Autodesk Inventor part; units mm, degrees
ref_plane "YZ Plane" through (0, 0, 0) normal (1, 0, 0) x (0, 1, 0)
ref_plane "XZ Plane" through (0, 0, 0) normal (0, 1, 0) x (-1, 0, 0)
ref_plane "XY Plane" through (0, 0, 0) normal (0, 0, 1) x (1, 0, 0)
sketch "Sketch1" plane through (0, 0, 0) normal (0, 0, 1) x (1, 0, 0)
  line L0 (0, 0) -> (600, 0)
  line L1 (100, -188) -> (500, -188)
  line L2 (500, -188) -> (500, -55)
  line L3 (500, -55) -> (600, -55)
  line L4 (600, -55) -> (600, 0)
  line L5 (100, -188) -> (100, -55)
  line L6 (0, -55) -> (0, 0)
  line L7 (0, -55) -> (100, -55)
  point P0 (300, -188)
  point P1 (300, 0)
  dimension "d0" = 600
  dimension "d1" = 188
  dimension "d2" = 400
  dimension "d3" = 133
extrude "Extrusion1" add sketch "Sketch1" along normal blind 10
sketch "Sketch2" plane through (0, 0, 10) normal (0, 0, 1) x (1, 0, 0)
  line L0 (600, 0) -> (0, 0)
  line L1 (500, -188) -> (100, -188)
  line L2 (600, 0) -> (300, 0)
  line L3 (300, 0) -> (300, -188)
  line L4 (300, -188) -> (600, -188)
  line L5 (600, -188) -> (600, 0)
extrude "Extrusion2" cut sketch "Sketch2" against normal through all
sketch "Sketch3" plane through (0, 0, 10) normal (0, 0, 1) x (1, 0, 0)
  circle A0 centre (10, -10) radius 2
  line L0 (300, 0) -> (0, 0)
  line L1 (0, 0) -> (0, -55)
  circle A1 centre (150, -10) radius 2
  circle A2 centre (290, -10) radius 2
  line L2 (300, -188) -> (300, 0)
  line L3 (10, -10) -> (290, -10) construction
  circle A3 centre (110, -178) radius 2
  line L4 (100, -55) -> (100, -188)
  line L5 (100, -188) -> (300, -188)
  circle A4 centre (290, -178) radius 2
  dimension "d8" = 4
  dimension "d9" = 10
  dimension "d10" = 10
  dimension "d11" = 4
  dimension "d12" = 4
  dimension "d13" = 10
  dimension "d14" = 4
  dimension "d15" = 10
  dimension "d16" = 10
  dimension "d17" = 4
  dimension "d18" = 10
  dimension "d19" = 10
extrude "Extrusion3" cut sketch "Sketch3" against normal through all
sketch "Sketch4" plane through (0, 0, 0) normal (0, 0, -1) x (-1, 0, 0)
  line L0 (-300, 0) -> (-300, -188)
  line L1 (-300, -32.5) -> (-318, -32.5)
  line L2 (-318, -32.5) -> (-318, -155.5)
  line L3 (-318, -155.5) -> (-300, -155.5)
  line L4 (-300, -155.5) -> (-300, -32.5)
  circle A0 centre (-310, -46.5) radius 2.5
  circle A1 centre (-310, -141.5) radius 2.5
  line L5 (-310, -46.5) -> (-310, -141.5) construction
  point P0 (0, 0)
  point P1 (-300, -94)
  point P2 (-310, -94)
  dimension "d22" = 18
  dimension "d23" = 123
  dimension "d24" = 5
  dimension "d25" = 5
  dimension "d26" = 10
  dimension "d27" = 95
extrude "Extrusion4" add sketch "Sketch4" against normal blind 5
properties part number "SP001b" material "ABS Plastic"
Read the model definition and answer for the solid it produces. Units are mm, in the model's axes. A direction names the side the tool comes from. Round coordinates to 2 decimals unless told otherwise and drop trailing zeros. Order: outer loops, then holes, each group sorted by start corner. A loop starts at its lowest first (then second) coordinate and runs counter-clockwise, first axis right, second up.
1) The part is cut by section C-C on x = 95.5. Write down the section's boundary in (y, z), plus the area to 3 significant figures.
2) The mould has two halves that part along X. Classify faces 1 (the face through (309, -93, 5)), 2 (the face through (0, -28, 5)): released by +X, released by -X, zero draft, split by the parting line, or undercut.
3) For faces 3 (the face through (181, -93, 10)), 4 (the face through (100, -122, 5)), determine the directions among +Z, -Z, +X, -X, +Y, -Y from which every point of the face is accessible in a straight line to the end or side of a thin tool.
4) Straight lines are drawn through the part: L1, parallel to Y at x = 310, z = 2.8; L2, parallel to X at y = -178, z = 3.75; L3, parallel to Y at x = 10, z = 4.75. For each, find the intervals that lie inside material, in ascending order.
5) The part is cut by section A-A on z = 8. Write down the section's boundary in (x, y), plus the area to 3 significant figures.
6) The part is cut by section D-D on y = -76. Write down the section's boundary in (x, z).
7) The part is cut by section B-B on y = -16. Write down the section's boundary in (x, z), plus the area to 3 significant figures.
8) Flat-ended cylindrical pins translate along their axes: pin 1 (9 mm diameter, centred on x = 308.5, y = -123.5, fed in from +Z); pin 2 (1.5 mm diameter, centred on x = 312, z = 2, fed in from +Y); pin 3 (5.5 mm diameter, centred on x = 313, z = 1.5, fed in from -Y). Find the tip coordinate at first contact, or state that the pin passes through.
Resolved:
1. outline: (-55, 0) - (0, 0) - (0, 10) - (-55, 10) - close
1. area: 550 mm2
2. face 1: zero draft
2. face 2: released by -X
3. face 3: +Z, +X, -X, +Y, -Y
3. face 4: +Z, -Z, -X, -Y
4. L1: y = -155.5 to -144, -139 to -49, -44 to -32.5
4. L2: x = 100 to 108, 112 to 288, 292 to 300
4. L3: y = -55 to -12, -8 to 0
5. outline: (0, -55) - (100, -55) - (100, -188) - (300, -188) - (300, 0) - (0, 0) - close; hole circle Ø4 at (10, -10); hole circle Ø4 at (110, -178); hole circle Ø4 at (150, -10); hole circle Ø4 at (290, -178); hole circle Ø4 at (290, -10)
5. area: 43,000 mm2
6. outline: (100, 0) - (318, 0) - (318, 5) - (300, 5) - (300, 10) - (100, 10) - close
7. outline: (0, 0) - (300, 0) - (300, 10) - (0, 10) - close
7. area: 3,000 mm2
8. pin 1: stops at z = 5
8. pin 2: stops at y = -32.5
8. pin 3: stops at y = -155.5
